Print and shaded views of the part. All mm, measured from the part's lowest x, y and z. Round coordinates to 2 decimals unless told otherwise and drop trailing zeros. Write each loop counter-clockwise with the first axis right and the second up, starting at its lowest first coordinate (ties: lowest second). Pieces come first, ordered by that corner, then holes. Notation, with made-up numbers: M 24.25,69.25 L 50.25,69.25 A9 cw 50.25,80.25 Z; hole C 53,63.5 d2. An arc over 180 degrees is marked long. Write item = value, one per line.
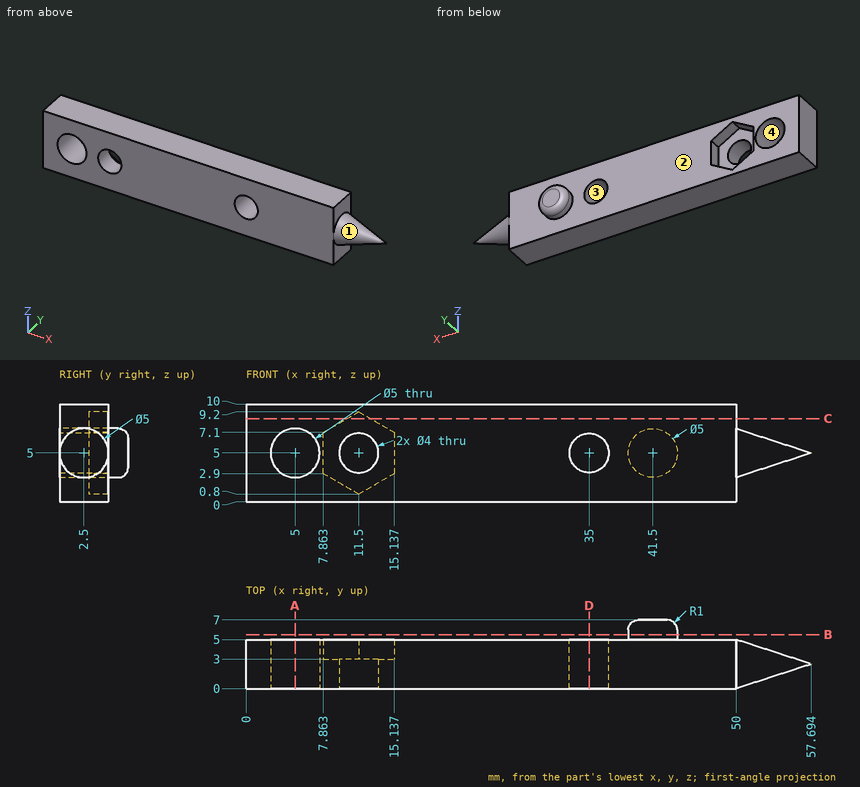
1. Probe probe 1 along Z at (x, y) = (3, 4.5); probe 2 along Y at (x, z) = (4.5, 1.75); probe 3 along Z at (x, y) = (4, 3.75). List the from-to ranges inside material, lowest first.
Responses:
probe_1 = 0 to 3.5, 6.5 to 10
probe_2 = 0 to 5
probe_3 = 0 to 2.71, 7.29 to 10
2. Band-saw the part on C-C (z = 8.5). List the corners of the cut face in (x, y).
Responses:
outline = M 0,0 L 50,0 L 50,5 L 12.71,5 L 12.71,3 L 10.29,3 L 10.29,5 L 0,5 Z
3. Band-saw the part on B-B (y = 5.5). List the corners of the cut face in (x, z).
Responses:
outline = C 41.5,5 d5
4. Mould opens along Z. For the marked faces 1, 2, 3 and 4 say: pulls with the +Z half, pulls with the -Z half, needs draft (parallel to the pull), parting line crosses it, or undercut.
Responses:
face_1 = parting line crosses it
face_2 = needs draft
face_3 = undercut
face_4 = undercut
5. Flat gauge pin, fed straight in: pin 1 (5 mm diameter, centred on x = 35, z = 5, fed in from +Y). Where does the tip first touch, or does it go through?
Responses:
pin_1 = 5
6. Band-saw the part on A-A (x = 5). List the corners of the cut face in (y, z), plus the area to 3 significant figures.
Responses:
outline = M 0,0 L 5,0 L 5,2.5 L 0,2.5 Z; M 0,7.5 L 5,7.5 L 5,10 L 0,10 Z
area = 25.0 mm²
7. Band-saw the part on D-D (x = 35). List the corners of the cut face in (y, z).
Responses:
outline = M 0,0 L 5,0 L 5,3 L 0,3 Z; M 0,7 L 5,7 L 5,10 L 0,10 Z
